Could you check a few things on this model? Use its own coordinates, in mm. Coordinates: 2 decimals unless noted, no trailing zeros. Order: outer loops, then holes, each group sorted by start corner. A loop starts at its lowest first (then second) coordinate and runs counter-clockwise, first axis right, second up. Notation, with made-up numbers: (46, 46.25) -> (70, 46.25) arc R24 cw to (70, 83.25) -> close; hole circle Ø9 at (14.5, -5). An arc over 180 degrees is marked (long way). Put each result on its own line as item: value. Start each with the question number.
Q1. We'd pull the mould along Y, two halves only. Please class faces 1 (the face through (50.089, -0.364, 5.275)), 2 (the face through (50, 21.641, 3)), 3 (the face through (50, 0, 17.293)): +Y half, -Y half, draft (parallel to the pull), parting line (faces both ways), or undercut.
Q2. If we section it at C-C (y = 0): Please give me the cut outline in (x, z).
Q3. Please list where these lines run through material, in increasing order: line 1 along Y through (x, z) = (22.5, 1.5); line 2 along Y through (x, z) = (19, -9.75); line 3 along Z through (x, y) = (95, -4).
Q4. If we section it at B-B (z = -3.75): Please give me the cut outline in (x, y).
Q5. If we section it at D-D (y = -13): Please give me the cut outline in (x, z).
Q6. If we section it at A-A (x = 86.5): Please give me the cut outline in (y, z), and give its area (3 significant figures).
Q7. Will this pin go through, and if not, where does the flat tip stop? pin 1 (4 mm diameter, centred on x = 22, y = 8.5, fed in from -Z).
from build123d import *

# Parameters (mm, degrees)
F1_DEPTH = 101.6


with BuildPart() as f1:
    # F0 (on Right) → F1 (new body)
    with BuildSketch(Plane.YZ):
        with BuildLine():
            ThreePointArc((-16.5608, -11.282155), (0, 5.278645), (16.5608, -11.282155))
            Line((16.5608, -11.282155), (21.6408, -11.282155))
            Line((21.6408, -11.282155), (21.6408, 17.292845))
            Line((21.6408, 17.292845), (-21.6408, 17.292845))
            Line((-21.6408, 17.292845), (-21.6408, -11.282155))
            Line((-21.6408, -11.282155), (-16.5608, -11.282155))
        make_face()
    extrude(amount=F1_DEPTH)


solid = f1.part
The answers:
1. face 1: undercut
1. face 2: +Y half
1. face 3: draft
2. outline: (0, 5.28) -> (101.6, 5.28) -> (101.6, 17.29) -> (0, 17.29) -> close
3. line 1: -21.64 to -10.53, 10.53 to 21.64
3. line 2: -21.64 to -16.49, 16.49 to 21.64
3. line 3: 4.79 to 17.29
4. outline: (0, -21.64) -> (101.6, -21.64) -> (101.6, -14.75) -> (0, -14.75) -> close; (0, 14.75) -> (101.6, 14.75) -> (101.6, 21.64) -> (0, 21.64) -> close
5. outline: (0, -1.02) -> (101.6, -1.02) -> (101.6, 17.29) -> (0, 17.29) -> close
6. outline: (-21.64, -11.28) -> (-16.56, -11.28) arc R16.56 cw to (16.56, -11.28) -> (21.64, -11.28) -> (21.64, 17.29) -> (-21.64, 17.29) -> close
6. area: 806 mm^2
7. pin 1: z = 1.52
